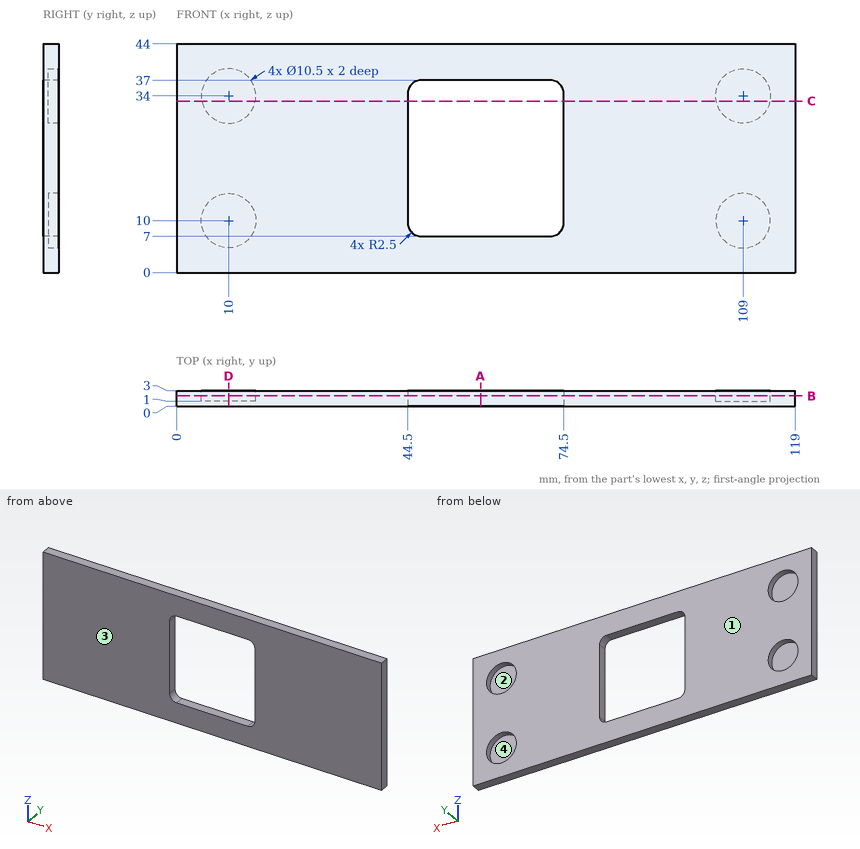
The figure shows three views and two pictorial views of one solid part (mm, origin at its lowest corner). Answer the questions. A direction names the side the tool comes from. Give positions to 0.01 mm unless a question says otherwise; leave off trailing zeros. Loops run counter-clockwise (first coordinate to the right, second up) from the corner with the lowest first, then second, coordinate; pieces in that order, holes last. Notation, with made-up numbers: (38.5, -6.75) - (63.5, -6.75) arc R19 ccw to (63.5, 11.25) - close; hole circle Ø7 at (-30.75, -9.5). An arc over 180 degrees is marked (long way). Answer in a Markdown table with one row per item.
(1) For a pull along X with two mould halves and no side action, classify the marked faces 1 and 2 as pulls with the +X half, pulls with the -X half, needs draft (parallel to the pull), parting line crosses it, or undercut.
Results list:
| item | result |
|---|---|
| face 1 | needs draft |
| face 2 | undercut |
(2) Flat-ended cylindrical pins translate along their axes: pin 1 Ø2 at (x, z) = (46, 22) entering from -Y; pin 2 Ø3 at (x, z) = (107, 35.5) entering from +Y. Find the tip coordinate at first contact, or state that the pin passes through.
Results list:
| item | result |
|---|---|
| pin 1 | passes through |
| pin 2 | stops at y = 1 |
(3) Section D-D (x = 10) is taken. Give the vertices of the cut face in (y, z).
Results list:
| item | result |
|---|---|
| outline | (0, 0) - (3, 0) - (3, 4.75) - (1, 4.75) - (1, 15.25) - (3, 15.25) - (3, 28.75) - (1, 28.75) - (1, 39.25) - (3, 39.25) - (3, 44) - (0, 44) - close |
(4) Section B-B (y = 2) is taken. Give the vertices of the cut face in (x, z).
Results list:
| item | result |
|---|---|
| outline | (0, 0) - (119, 0) - (119, 44) - (0, 44) - close; hole circle Ø10.5 at (10, 10); hole circle Ø10.5 at (10, 34); hole (44.5, 9.5) arc R2.5 ccw to (47, 7) - (72, 7) arc R2.5 ccw to (74.5, 9.5) - (74.5, 34.5) arc R2.5 ccw to (72, 37) - (47, 37) arc R2.5 ccw to (44.5, 34.5) - close; hole circle Ø10.5 at (109, 10); hole circle Ø10.5 at (109, 34) |
(5) Section A-A (x = 58.5) is taken. Give the vertices of the cut face in (y, z).
Results list:
| item | result |
|---|---|
| outline | (0, 0) - (3, 0) - (3, 7) - (0, 7) - close; (0, 37) - (3, 37) - (3, 44) - (0, 44) - close |
(6) Section C-C (z = 33) is taken. Give the vertices of the cut face in (x, y).
Results list:
| item | result |
|---|---|
| outline | (0, 0) - (44.5, 0) - (44.5, 3) - (15.15, 3) - (15.15, 1) - (4.85, 1) - (4.85, 3) - (0, 3) - close; (74.5, 0) - (119, 0) - (119, 3) - (114.15, 3) - (114.15, 1) - (103.85, 1) - (103.85, 3) - (74.5, 3) - close |
(7) Consider L1, parallel to X at y = 1.5, z = 34; L2, parallel to Z at x = 109, y = 2.3; L3, parallel to X at y = 0.9, z = 30.5. Determine where each line is inside the solid, lowest interval first. Write a range as [from, to].
Results list:
| item | result |
|---|---|
| L1 | x = [0, 4.75], [15.25, 44.5], [74.5, 103.75], [114.25, 119] |
| L2 | z = [0, 4.75], [15.25, 28.75], [39.25, 44] |
| L3 | x = [0, 44.5], [74.5, 119] |
(8) A tool of negligible diameter and unlimited length cuts with its end or side. For the marked faces 3 and 4, from which of +Z, -Z, +X, -X, +Y, -Y can it reach the whole face along a straight path? Write none if from no direction.
Results list:
| item | result |
|---|---|
| face 3 | +Z, -Z, +X, -X, -Y |
| face 4 | +Y |
